```python
from build123d import *

# Parameters (mm, degrees)
SKETCH_1_R               = 28.5
EXTRUDE_1_DEPTH          = 10
SKETCH_36_R              = 3.85
EXTRUDE_5_DEPTH          = 5
PATTERN_CIRCULAR_4_COUNT = 8
SKETCH_42_R              = 39.215237935
SKETCH_42_R_2            = 28.25
CUT_EXTRUDE_1_DEPTH      = 44.005813698
HOLE_WIZARD_M2_3_D       = 2.4


with BuildPart() as part:
    # 스케치1 → 보스-돌출1 (new body)
    with BuildSketch(Plane(origin=(0, 0, 0), x_dir=(1, 0, 0), z_dir=(0, 1, 0))):
        with Locations(Location((0, 0, 0), (0, 0, 270))):
            Circle(SKETCH_1_R)
    extrude(amount=EXTRUDE_1_DEPTH)

    # 스케치36 → 보스-돌출5 (add)
    with BuildSketch(Plane.XZ):
        with Locations(Location((0, 14.33, 0), (0, 0, 90))):
            Circle(SKETCH_36_R)
        with Locations(Location((12.410144036, -7.165, 0), (0, 0, 90))):
            Circle(SKETCH_36_R)
        with Locations(Location((-12.410144036, -7.165, 0), (0, 0, 90))):
            Circle(SKETCH_36_R)
    extrude(amount=EXTRUDE_5_DEPTH)

    # 스케치41 → M2 여유 구멍1 (revolve, cut)
    with BuildSketch(Plane(origin=(-28.5, 5, 0), x_dir=(0, 0, 1), z_dir=(0, 1, 0))):
        Polygon((0, 0), (0, 15.721032743), (1.2, 15), (1.2, 0), align=None)
    hole_wizard_m2_1 = revolve(axis=Axis((-34.85, 5, 0), (1, 0, 0)), mode=Mode.SUBTRACT)

    # 원형 패턴4: M2 여유 구멍1 ×8 about axis
    pattern_circular_4_axis = Axis((0, 10, 0), (0, 1, 0))
    for i in range(1, PATTERN_CIRCULAR_4_COUNT):
        add(hole_wizard_m2_1.rotate(pattern_circular_4_axis, i * 360 / PATTERN_CIRCULAR_4_COUNT), mode=Mode.SUBTRACT)

    # 스케치42 → 컷-돌출1 (cut, through all)
    with BuildSketch(Plane(origin=(0, 10, 0), x_dir=(1, 0, 0), z_dir=(0, 1, 0))):
        Circle(SKETCH_42_R)
        with Locations(Location((0, 0, 0), (0, 0, 270))):
            Circle(SKETCH_42_R_2, mode=Mode.SUBTRACT)
    extrude(amount=-CUT_EXTRUDE_1_DEPTH, mode=Mode.SUBTRACT)

    # M2 여유 구멍3 (through all)
    with Locations(Plane(origin=(0, 0, 0), x_dir=(-1, 0, 0), z_dir=(0, -1, 0))):
        with Locations((-12.410144036, -7.165), (0, 14.33), (12.410144036, -7.165)):
            Hole(HOLE_WIZARD_M2_3_D / 2)


solid = part.part
```
Can you work these out from the model? Positions are in its coordinate system, mm. A direction names the side the tool comes from. Round coordinates to 2 decimals unless told otherwise and drop trailing zeros. Loops run counter-clockwise (first coordinate to the right, second up) from the corner with the lowest first, then second, coordinate; pieces in that order, holes last. Notation, with made-up numbers: M -34.75,85 L 17.25,85 A28 ccw 17.25,109 Z; hole C -27.5,50.25 d4. An arc over 180 degrees is marked long. Answer as a JSON object with one key per item and string values. Group by question number.
Q1. Imagine slicing it at C-C, the plane z = -12. Count the separate pieces of the cut face and the enclosed holes in it, then the cut area to 3 significant figures.
Q2. On a 3-axis mill with a long thin cutter (end or side, diameter ignored), from which of +Z, -Z, +X, -X, +Y, -Y can I reach the whole of each face in a straight line? I mean faces 5 (the cylindrical face through (1.2, 4.95, -21.39)), 6 (the conical face through (9.016, 4.859, 9.233)), 7 (the flat face through (0, 0, 0)). Say none if no direction works.
Q3. Will these pins go through, and if not, where does the flat tip stop? pin 1 (1.9 mm diameter, centred on y = 5, z = 0, fed in from +X); pin 2 (1.5 mm diameter, centred on x = -13, y = 3, fed in from -Z); pin 3 (5 mm diameter, centred on y = 3, z = -18.5, fed in from -X).
Q4. Imagine slicing it at B-B, the plane x = -7. Please give me the cut outline in (y, z).
Q5. Please list where these lines run through material, in increasing order: L1, parallel to Z at x = 0, y = 2.45; L2, parallel to Y at x = 0, z = -21; L3, parallel to X at y = 6.25, z = 8.
Q6. Imagine slicing it at A-A, the plane y = 8.5. Please give me the cut outline in (x, z) (3 decimals), then the cut area to 3 significant figures.
Q7. We'd pull the mould along Y, two halves only. Please class faces 1 (the cylindrical face through (15.29, 3.988, 14.378)), 2 (the cylindrical face through (14.75, -2.46, -10.22)), 3 (the flat face through (-12, -5, -7)), 4 (the flat face through (0, 10, 0)): +Y half, -Y half, draft (parallel to the pull), parting line (faces both ways), or undercut.
Findings:
{
 "1": {"separate pieces": "1", "enclosed holes": "2", "area": "499 mm2"},
 "2": {"face 5": "-Z", "face 6": "none", "face 7": "-Y"},
 "3": {"pin 1": "stops at x = 13.35", "pin 2": "stops at z = -25.46", "pin 3": "stops at x = -23.28"},
 "4": {"outline": "M 0,-27.37 L 10,-27.37 L 10,27.37 L 0,27.37 Z"},
 "5": {"L1": "z = -28.25 to -15.53, -13.13 to 28.25", "L2": "y = 0 to 3.8, 6.2 to 10", "L3": "x = -27.09 to -13.27, -11.55 to 11.55, 13.27 to 27.09"},
 "6": {"outline": "C 0,0 d56.5; hole C -12.41,7.165 d2.4; hole C 0,-14.33 d2.4; hole C 12.41,7.165 d2.4", "area": "2,490 mm2"},
 "7": {"face 1": "undercut", "face 2": "draft", "face 3": "-Y half", "face 4": "+Y half"}
}
